from build123d import *

# Parameters (mm, degrees)
SKETCH1_R                      = 76
BOSS_EXTRUDE1_DEPTH            = 5.6
F_8_0_199_DIAMETER_HOLE1_D     = 5.0546
F_8_0_199_DIAMETER_HOLE1_DEPTH = 8.481444958
F_8_0_199_DIAMETER_HOLE1_TIP   = 1.518555042


with BuildPart() as part:
    # Sketch1 → Boss-Extrude1 (new body)
    with BuildSketch(Plane.XY):
        Circle(SKETCH1_R)
    extrude(amount=BOSS_EXTRUDE1_DEPTH)

    # #8 (0.199) Diameter Hole1
    with Locations(Plane(origin=(0, 0, 0), x_dir=(-1, 0, 0), z_dir=(0, 0, -1))):
        with Locations((-50.478019657, 50.478019657), (0, 71.3867), (50.478019657, 50.478019657), (71.3867, 0), (50.478019657, -50.478019657), (0, -71.3867), (-50.478019657, -50.478019657), (-71.3867, 0)):
            Hole(F_8_0_199_DIAMETER_HOLE1_D / 2, depth=F_8_0_199_DIAMETER_HOLE1_DEPTH)
            with Locations((0, 0, -(F_8_0_199_DIAMETER_HOLE1_DEPTH + F_8_0_199_DIAMETER_HOLE1_TIP / 2))):  # 118° drill point
                Cone(0, F_8_0_199_DIAMETER_HOLE1_D / 2, F_8_0_199_DIAMETER_HOLE1_TIP, mode=Mode.SUBTRACT)


solid = part.part
Read the model definition and answer for the solid it produces. Units are mm, in the model's axes. Give positions to 0.01 mm unless a question says otherwise; leave off trailing zeros. Loops run counter-clockwise (first coordinate to the right, second up) from the corner with the lowest first, then second, coordinate; pieces in that order, holes last. Notation, with made-up numbers: (13.5, 86) -> (58.5, 86) arc R26 ccw to (58.5, 107) -> close; hole circle Ø11 at (27.5, -40). An arc over 180 degrees is marked (long way). Answer as CSV lines item,"result".
Item 1: Find section C-C on z = 1.5. State how many separate pieces and enclosed holes the cut face has, plus the area to 3 significant figures.
Returned:
separate pieces,"1"
enclosed holes,"8"
area,"18,000 mm²"
Item 2: Find section A-A on y = 0. Give the vertices of the cut face in (x, z), plus the area to 3 significant figures.
Returned:
outline,"(-76, 0) -> (-73.91, 0) -> (-73.91, 5.6) -> (-76, 5.6) -> close; (-68.86, 0) -> (68.86, 0) -> (68.86, 5.6) -> (-68.86, 5.6) -> close; (73.91, 0) -> (76, 0) -> (76, 5.6) -> (73.91, 5.6) -> close"
area,"795 mm²"
Item 3: Find section D-D on x = -56. Give the vertices of the cut face in (y, z).
Returned:
outline,"(-51.38, 0) -> (51.38, 0) -> (51.38, 5.6) -> (-51.38, 5.6) -> close"
Item 4: Each of these flat-tipped pins is pushed along its axis until it touches: pin 1 (4.5 mm diameter, centred on x = 0, y = -71.39, fed in from +Z); pin 2 (2 mm diameter, centred on x = 37.5, z = 3, fed in from -Y). Where does it stop, or does it pass through?
Returned:
pin 1,"passes through"
pin 2,"stops at y = -66.66"
Item 5: Determine the mould class of faces 1 (the face through (35.069, -67.425, 2.761)), 2 (the face through (-1, 1, 5.6)), 3 (the face through (52.9, 51.2, 2.8)) for opening direction Y: +Y half, -Y half, draft (parallel to the pull), parting line (faces both ways), or undercut.
Returned:
face 1,"parting line"
face 2,"draft"
face 3,"undercut"
Item 6: Consider line 1 (Y direction, x = 0, z = 1.85); line 2 (Y direction, x = 52.5, z = 2.35); line 3 (X direction, y = -49.5, z = 2.45). Determine where each line is inside the solid, lowest interval first. Write a range as [from, to].
Returned:
line 1,"y = [-76, -73.91], [-68.86, 68.86], [73.91, 76]"
line 2,"y = [-54.95, -51.99], [-48.96, 48.96], [51.99, 54.95]"
line 3,"x = [-57.67, -52.81], [-48.15, 48.15], [52.81, 57.67]"
